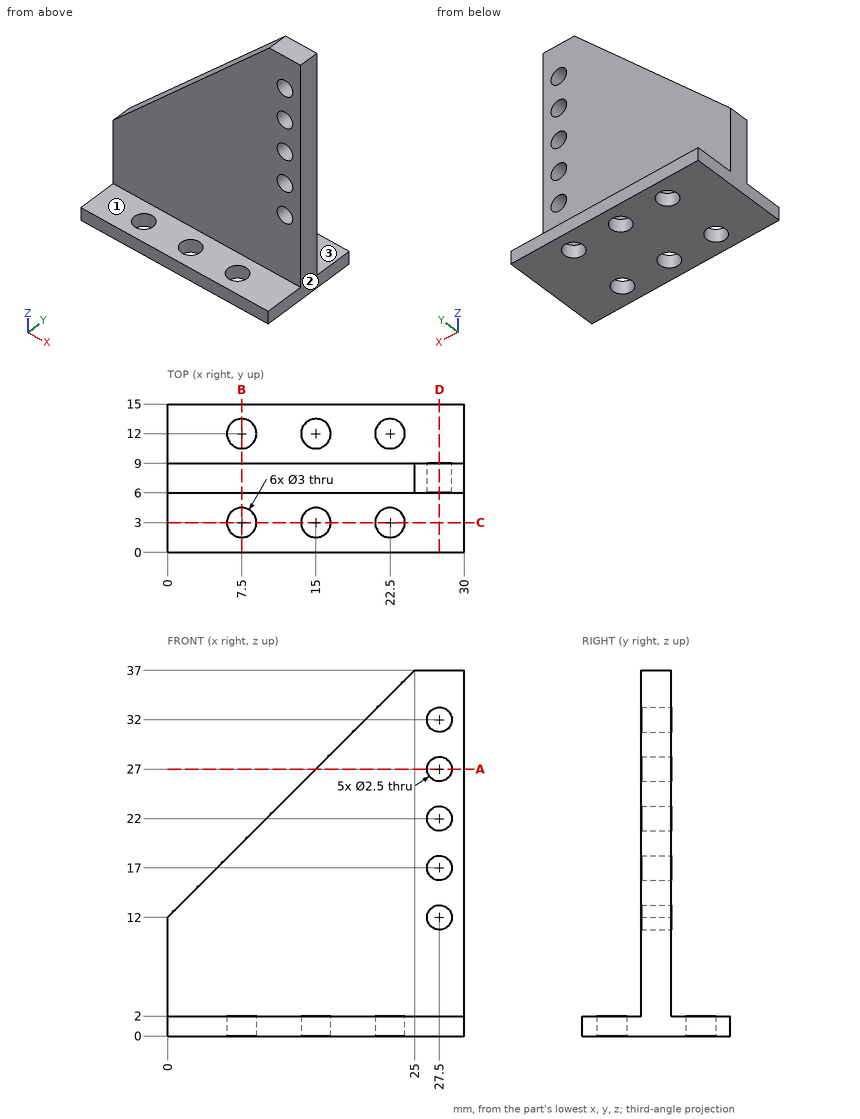
Source: three-view drawing plus pictorial views. Frame: mm from the lowest corner of the part. A direction names the side the tool comes from. Coordinates: 2 decimals unless noted, no trailing zeros. Order: outer loops, then holes, each group sorted by start corner. A loop starts at its lowest first (then second) coordinate and runs counter-clockwise, first axis right, second up. Notation, with made-up numbers: M 44,17.25 L 90,17.25 A20 ccw 90,32.25 Z; hole C 45,-13.75 d9. An arc over 180 degrees is marked long. One line per question, with ' | ' between items. Start each with the question number.
Item 1: Set-up query: the marked faces 1, 2 and 3. Return all of +Z, -Z, +X, -X, +Y, -Y with unobstructed straight access to the full face (end or side cutting, diameter ignored); none if empty.
Item 2: Cut plane B-B, the plane x = 7.5. Return the cut outline in (y, z), then the cut area to 3 significant figures.
Item 3: Cut plane D-D, the plane x = 27.5. Return the cut outline in (y, z), then the cut area to 3 significant figures.
Item 4: Pin query (flat end, axial travel): pin 1 Ø1.8 at (x, y) = (20.5, 13) entering from +Z; pin 2 Ø2 at (x, z) = (27.5, 27) entering from -Y; pin 3 Ø1 at (x, y) = (3.5, 7.5) entering from +Z; pin 4 Ø4 at (x, z) = (27.5, 17) entering from -Y. Return the tip coordinate at first contact, or that it passes through.
Item 5: Cut plane A-A, the plane z = 27. Return the cut outline in (x, y).
Item 6: Ray query, probe 1 along Z at (x, y) = (27.5, 6.7); probe 2 along Y at (x, z) = (22.5, 1.55); probe 3 along Z at (x, y) = (12.5, 14). Return the intervals inside material, ascending. Write a range as [from, to].
Item 7: Cut plane C-C, the plane y = 3. Return the cut outline in (x, z).
A:
1) face 1: +Z, +X, -X, -Y | face 2: +Z, -Z, +X, +Y, -Y | face 3: +Z, +X, -X, +Y
2) outline: M 0,0 L 1.5,0 L 1.5,2 L 0,2 Z; M 4.5,0 L 10.5,0 L 10.5,2 L 9,2 L 9,19.5 L 6,19.5 L 6,2 L 4.5,2 Z; M 13.5,0 L 15,0 L 15,2 L 13.5,2 Z | area: 70.5 mm2
3) outline: M 0,0 L 15,0 L 15,2 L 9,2 L 9,10.75 L 6,10.75 L 6,2 L 0,2 Z; M 6,13.25 L 9,13.25 L 9,15.75 L 6,15.75 Z; M 6,18.25 L 9,18.25 L 9,20.75 L 6,20.75 Z; M 6,23.25 L 9,23.25 L 9,25.75 L 6,25.75 Z; M 6,28.25 L 9,28.25 L 9,30.75 L 6,30.75 Z; M 6,33.25 L 9,33.25 L 9,37 L 6,37 Z | area: 97.5 mm2
4) pin 1: stops at z = 2 | pin 2: passes through | pin 3: stops at z = 16 | pin 4: stops at y = 6
5) outline: M 15,6 L 26.25,6 L 26.25,9 L 15,9 Z; M 28.75,6 L 30,6 L 30,9 L 28.75,9 Z
6) probe 1: z = [0, 10.75], [13.25, 15.75], [18.25, 20.75], [23.25, 25.75], [28.25, 30.75], [33.25, 37] | probe 2: y = [0, 1.5], [4.5, 10.5], [13.5, 15] | probe 3: z = [0, 2]
7) outline: M 0,0 L 6,0 L 6,2 L 0,2 Z; M 9,0 L 13.5,0 L 13.5,2 L 9,2 Z; M 16.5,0 L 21,0 L 21,2 L 16.5,2 Z; M 24,0 L 30,0 L 30,2 L 24,2 Z
